Build history of the part. All positions in model axes, mm. A direction names the side the tool comes from. Give positions to 0.01 mm unless a question says otherwise; leave off trailing zeros. Order: outer loops, then holes, each group sorted by start corner. A loop starts at its lowest first (then second) coordinate and runs counter-clockwise, first axis right, second up. Notation, with made-up numbers: (63.25, 72.5) - (67.25, 72.5) arc R32 cw to (67.25, 105.5) - close; hole circle Ø10 at (68.25, 25). An arc over 180 degrees is marked (long way). Write each question's results on one line, items separated by ' | '. Start each with the question number.
1) Two-plate mould, pull along X, no slides. Class faces 1 (the face through (-49.096, 345, 29)), 2 (the face through (-33, 700, 32)), 3 (the face through (-33, 345, 20)), 4 (the face through (-17, 345, 32)): +X half, -X half, draft (parallel to the pull), parting line (faces both ways), or undercut.
2) Tool access for faces 5 (the face through (-33, 345, 40)), 6 (the face through (-47.096, 345, 29)): list every direction of +Z, -Z, +X, -X, +Y, -Y with a clear straight run to the whole face (end or side of a thin tool).
3) Drill centre lines: line 1 along X through (y, z) = (92, 32.25); line 2 along Z through (x, y) = (-26, 443); line 3 along X through (y, z) = (362.5, 21.5). Where is each one in solid material? Low to high. Write a range as from..to.
4) Cut at B-B on y = 298. List the corners of the cut face in (x, z), plus the area to 3 significant figures.
5) Cut at A-A on x = -39.5. List the corners of the cut face in (y, z), plus the area to 3 significant figures.
from build123d import *

# Parameters (mm, degrees)
F2_DEPTH = 1910
F7_DEPTH = 700
F9_DEPTH = 2000


with BuildPart() as f2:
    # F1 (on Front) → F2 (new body)
    with BuildSketch(Plane.XZ):
        with BuildLine():
            Line((7.5, 37.974085065), (7.5, 40))
            Line((7.5, 40), (-15, 40))
            Line((-15, 40), (-15, 37))
            Line((-15, 37), (-15, 31))
            Line((-15, 31), (-15, 29))
            Line((-15, 29), (-15, 26))
            Line((-15, 26), (-15, 24))
            Line((-15, 24), (-13, 24))
            Line((-13, 24), (-11, 24))
            Line((-11, 24), (-11, 26))
            Line((-11, 26), (-9, 26))
            Line((-9, 26), (-9, 20))
            Line((-9, 20), (-11, 20))
            Line((-11, 20), (-11, 22))
            Line((-11, 22), (-15, 22))
            Line((-15, 22), (-15, 18))
            Line((-15, 18), (-15, 7.7))
            Line((-15, 7.7), (-13, 7.7))
            Line((-13, 7.7), (-13, 11.4920835048))
            Line((-13, 11.4920835048), (-7, 11.4920835048))
            Line((-7, 11.4920835048), (-7, 3.7))
            Line((-7, 3.7), (-11, 3.7))
            Line((-11, 3.7), (-11, 5.7))
            Line((-11, 5.7), (-15, 5.7))
            Line((-15, 5.7), (-15, 3))
            Line((-15, 3), (-15, 0))
            Line((-15, 0), (-13, 0))
            Line((-13, 0), (-12, 0))
            Line((-12, 0), (-5, 0))
            Line((-5, 0), (-5, 13.4920835048))
            Line((-5, 13.4920835048), (-7, 13.4920835048))
            Line((-7, 13.4920835048), (-9.1588944197, 13.4920835048))
            Line((-9.1588944197, 13.4920835048), (-9.1588944197, 15.4920835048))
            Line((-9.1588944197, 15.4920835048), (1.5, 20))
            Line((1.5, 20), (10.8411055803, 15.4920835048))
            Line((10.8411055803, 15.4920835048), (10.8411055803, 13.4920835048))
            Line((10.8411055803, 13.4920835048), (8, 13.4920835048))
            Line((8, 13.4920835048), (8, 0))
            Line((8, 0), (17, 0))
            Line((17, 0), (17, 40))
            Line((17, 40), (8.5, 40))
            Line((8.5, 40), (8.5, 37.974085065))
            ThreePointArc((8.5, 37.974085065), (11.5604089792, 36.6859489396), (13.3185590744, 33.8691589154))
            Line((13.3185590744, 33.8691589154), (13.4318527537, 31.7073867348))
            ThreePointArc((13.4318527537, 31.7073867348), (4.0126863822, 28.7323088758), (7.5, 37.974085065))
        make_face()
        Polygon((-8.3634709733, 18), (-11.1588944197, 16.817744602), (-11.1588944197, 15.4920835048), (-11.1588944197, 13.4920835048), (-13, 13.4920835048), (-13, 18), align=None, mode=Mode.SUBTRACT)
        with BuildLine():
            Line((-13, 34), (-13, 37.9999987781))
            Line((-13, 37.9999987781), (2.9081163149, 37.9999987781))
            ThreePointArc((2.9081163149, 37.9999987781), (3.810445381, 26.2974906682), (15, 29.8410427327))
            Line((15, 29.8410427327), (15, 2))
            Line((15, 2), (10, 2))
            Line((10, 2), (10, 12))
            Line((10, 12), (12.8411055803, 12))
            Line((12.8411055803, 12), (12.8411055803, 16.7476188273))
            Line((12.8411055803, 16.7476188273), (1.5543358685, 22.194491783))
            Line((1.5543358685, 22.194491783), (-7, 18.5766464184))
            Line((-7, 18.5766464184), (-7, 28))
            Line((-7, 28), (-13, 28))
            Line((-13, 28), (-13, 34))
        make_face(mode=Mode.SUBTRACT)
        with BuildLine():
            Line((13.0918836851, 37.9999987781), (13.1020709306, 37.9999987781))
            Line((13.1020709306, 37.9999987781), (13.1025921338, 37.9900536295))
            ThreePointArc((13.1025921338, 37.9900536295), (13.0972403349, 37.9950288154), (13.0918836851, 37.9999987781))
        make_face(mode=Mode.SUBTRACT)
    extrude(amount=-F2_DEPTH)

    # F8 (on face) → F9 (cut)
    with BuildSketch(Plane.XZ):
        Polygon((17, 0), (17, 40), (-15, 40), (-15, 3), (-15, 0), align=None)
    extrude(amount=-F9_DEPTH, mode=Mode.SUBTRACT)


with BuildPart() as f7:
    # F6 (on face) → F7 (new body)
    with BuildSketch(Plane.XZ):
        with BuildLine():
            Line((-17.7814291848, 40), (-25.5, 40))
            Line((-25.5, 40), (-49.096, 40))
            Line((-49.096, 40), (-49.096, 18))
            Line((-49.096, 18), (-17, 18))
            Line((-17, 18), (-17, 22))
            Line((-17, 22), (-19, 22))
            Line((-19, 22), (-19, 20))
            Line((-19, 20), (-47.096, 20))
            Line((-47.096, 20), (-47.096, 38))
            Line((-47.096, 38), (-31.0964418097, 38))
            ThreePointArc((-31.0964418097, 38), (-30.1932729017, 26.2962600635), (-19, 29.8323432536))
            Line((-19, 29.8323432536), (-19, 24))
            Line((-19, 24), (-17, 24))
            Line((-17, 24), (-17, 39.349379475))
            Line((-17, 39.349379475), (-21.4759115093, 35.6227207421))
            ThreePointArc((-21.4759115093, 35.6227207421), (-30.2216849679, 28.9915813466), (-22.1157647548, 36.3912178626))
            Line((-22.1157647548, 36.3912178626), (-17.7814291848, 40))
        make_face()
    extrude(amount=-F7_DEPTH)


solid = f7.part
Results:
1) face 1: -X half | face 2: draft | face 3: undercut | face 4: +X half
2) face 5: +Z, +X, -X, +Y, -Y | face 6: +Y, -Y
3) line 1: -49.1..-47.1, -33.49..-31.49, -20.51..-17 | line 2: 18..20, 25.01..27.01, 38..40 | line 3: -49.1..-47.1, -19..-17
4) outline: (-49.1, 18) - (-17, 18) - (-17, 22) - (-19, 22) - (-19, 20) - (-47.1, 20) - (-47.1, 38) - (-31.1, 38) arc R7.49 ccw (long way) to (-19, 29.83) - (-19, 24) - (-17, 24) - (-17, 39.35) - (-21.48, 35.62) arc R5.49 cw (long way) to (-22.12, 36.39) - (-17.78, 40) - (-49.1, 40) - close | area: 258 mm^2
5) outline: (0, 18) - (700, 18) - (700, 20) - (0, 20) - close; (0, 38) - (700, 38) - (700, 40) - (0, 40) - close | area: 2,800 mm^2
